Source: CAD feature listing. Evaluate the final solid. Frame: model axes, mm. A direction names the side the tool comes from. Give positions to 0.01 mm unless a question says otherwise; leave off trailing zeros. Loops run counter-clockwise (first coordinate to the right, second up) from the corner with the lowest first, then second, coordinate; pieces in that order, holes last. Notation, with made-up numbers: M 87.5,37.5 L 110.5,37.5 A35 ccw 110.5,73.5 Z; hole C 13,1 d3. An arc over 180 degrees is marked long. Answer in a Markdown table with one row per item.
```python
from build123d import *

# Parameters (mm, degrees)
SKETCH1_R             = 3.9
BOSS_EXTRUDE1_DEPTH   = 29.5
SKETCH2_R             = 6.75
BOSS_EXTRUDE2_DEPTH   = 3
SKETCH3_R             = 4.5
FILLET1_R             = 0.5
CUT_EXTRUDE1_DEPTH    = 2.1
M6_TAPPED_HOLE1_D     = 5
M6_TAPPED_HOLE1_DEPTH = 15
M6_TAPPED_HOLE1_TIP   = 1.502151548
CHAMFER1_SIZE         = 0.15


with BuildPart() as part:
    # Sketch1 → Boss-Extrude1 (new body)
    with BuildSketch(Plane.XY):
        Circle(SKETCH1_R)
    extrude(amount=BOSS_EXTRUDE1_DEPTH)

    # Sketch2 → Boss-Extrude2 (add)
    with BuildSketch(Plane.XY.offset(29.5)):
        Circle(SKETCH2_R)
    extrude(amount=BOSS_EXTRUDE2_DEPTH)

    # Sketch3 → section 1 of loft1
    with BuildSketch(Plane.XY.offset(36), mode=Mode.PRIVATE) as loft1_s1:
        Circle(SKETCH3_R)
    # loft up to a face of the part (loft1)
    loft([Face(Wire([part.edges().sort_by_distance((-4.620692965, 4.920538235, 32.5))[0]])), loft1_s1.sketch])

    # Fillet1
    fillet1_edges = [part.edges().sort_by_distance(p)[0] for p in [
        (-6.75, 0, 29.5),
        (-6.75, 0, 32.5),
        (-4.5, 0, 36),
    ]]
    fillet(fillet1_edges, radius=FILLET1_R)

    # Sketch6 → Cut-Extrude1 (cut)
    with BuildSketch(Plane.XY.offset(36)):
        Polygon((1.533242561, -0.412311271), (1.123693315, 1.121671372), (-0.409549246, 1.533982643), (-1.533242561, 0.412311271), (-1.123693315, -1.121671372), (0.409549246, -1.533982643), align=None)
    extrude(amount=-CUT_EXTRUDE1_DEPTH, mode=Mode.SUBTRACT)

    # M6 Tapped Hole1
    with Locations(Plane(origin=(0, 0, 0), x_dir=(-1, 0, 0), z_dir=(0, 0, -1))):
        with Locations((0, 0)):
            Hole(M6_TAPPED_HOLE1_D / 2, depth=M6_TAPPED_HOLE1_DEPTH)
            with Locations((0, 0, -(M6_TAPPED_HOLE1_DEPTH + M6_TAPPED_HOLE1_TIP / 2))):  # 118° drill point
                Cone(0, M6_TAPPED_HOLE1_D / 2, M6_TAPPED_HOLE1_TIP, mode=Mode.SUBTRACT)

    # Chamfer1
    chamfer1_edges = [part.edges().sort_by_distance(p)[0] for p in [
        (-3.9, 0, 0),
    ]]
    chamfer(chamfer1_edges, length=CHAMFER1_SIZE)


solid = part.part
```
Q1. Ray query, probe 1 along Y at (x, z) = (0, 12.25); probe 2 along Z at (x, y) = (-4, -1); probe 3 along Y at (x, z) = (-1.75, 6). Return the intervals inside material, ascending. Write a range as from..to.
Values follow:
| item | result |
|---|---|
| probe 1 | -3.9..-2.5, 2.5..3.9 |
| probe 2 | 29.5..36 |
| probe 3 | -3.49..-1.79, 1.79..3.49 |
Q2. Section query B-B (z = 19). Output: boundary loops of the cut face in (x, y).
Values follow:
| item | result |
|---|---|
| outline | C 0,0 d7.8 |
Q3. Contact query for flat-ended pins moving along their axis: pin 1 Ø6 at (y, z) = (-1, 10.5) entering from +X; pin 2 Ø2 at (x, y) = (4.5, -0.5) entering from -Z; pin 3 Ø4 at (y, z) = (-3.5, 20.5) entering from +X; pin 4 Ø1 at (y, z) = (-3, 10.5) entering from -X. Output: stop coordinate, or through.
Values follow:
| item | result |
|---|---|
| pin 1 | x = 3.9 |
| pin 2 | z = 0 |
| pin 3 | x = 3.6 |
| pin 4 | x = -2.99 |
Q4. Section query A-A (z = 8). Output: boundary loops of the cut face in (x, y), plus the area to 3 significant figures.
Values follow:
| item | result |
|---|---|
| outline | C 0,0 d7.8; hole C 0,0 d5 |
| area | 28.1 mm^2 |
Q5. Mould query, pull axis X, two halves, no side actions, for faces 1 (the cylindrical face through (-1.46, -6.59, 31.16)), 2 (the flat face through (-3, -3, 29.5)), 3 (the flat face through (0, 0, 33.9)). Classes: +X half, -X half, draft (parallel to the pull), parting line (faces both ways), or undercut.
Values follow:
| item | result |
|---|---|
| face 1 | parting line |
| face 2 | draft |
| face 3 | undercut |
Q6. Section query C-C (z = 33.5). Output: boundary loops of the cut face in (x, y).
Values follow:
| item | result |
|---|---|
| outline | C 0,0 d12.21 |
Q7. Reachability of faces 4 (the cylindrical face through (-2.87, 2.64, 14.62)), 5 (the flat face through (0.964, -0.981, 34.965)), 6 (the flat face through (0, 3, 0)) from +Z, -Z, +X, -X, +Y, -Y: full face, straight path, thin tool, end or side. Return the list, or none.
Values follow:
| item | result |
|---|---|
| face 4 | -Z |
| face 5 | +Z |
| face 6 | -Z, +X, -X, +Y, -Y |
